Autodesk Inventor part; units mm, degrees
ref_plane "YZ Plane" through (0, 0, 0) normal (1, 0, 0) x (0, 1, 0)
ref_plane "XZ Plane" through (0, 0, 0) normal (0, 1, 0) x (-1, 0, 0)
ref_plane "XY Plane" through (0, 0, 0) normal (0, 0, 1) x (1, 0, 0)
sketch "Sketch1" plane through (0, 0, 0) normal (0, 1, 0) x (-1, 0, 0)
  circle A0 centre (0, 0) radius 6.65
  dimension "d0" = 13.3
extrude "Extrusion1" add sketch "Sketch1" along normal blind 13.3
sketch "Sketch2" plane through (0, 13.3, 0) normal (0, 1, 0) x (1, 0, 0)
  line L0 (0, 10.65) -> (9.2232, 5.325)
  line L1 (9.2232, 5.325) -> (9.2232, -5.325)
  line L2 (9.2232, -5.325) -> (0, -10.65)
  line L3 (0, -10.65) -> (-9.2232, -5.325)
  line L4 (-9.2232, -5.325) -> (-9.2232, 5.325)
  line L5 (-9.2232, 5.325) -> (0, 10.65)
  point P0 (0, 0)
  point P1 (0, 0)
extrude "Extrusion2" add sketch "Sketch2" along normal blind 12.4
sketch "Sketch3" plane through (0, 25.7, 0) normal (0, 1, 0) x (1, 0, 0)
  circle A0 centre (0, 0) radius 11.9
  dimension "d6" = 23.8
extrude "Extrusion3" add sketch "Sketch3" along normal blind 13
sketch "Sketch4" plane through (0, 38.7, 0) normal (0, 1, 0) x (1, 0, 0)
  circle A0 centre (0, 0) radius 11
  dimension "d9" = 22
extrude "Extrusion4" add sketch "Sketch4" along normal blind 1.7
sketch "Sketch5" plane through (0, 40.4, 0) normal (0, 1, 0) x (1, 0, 0)
  circle A0 centre (0, 0) radius 11.9
extrude "Extrusion5" add sketch "Sketch5" along normal blind 4.2
sketch "Sketch6" plane through (0, 44.6, 0) normal (0, 1, 0) x (1, 0, 0)
  circle A0 centre (0, 0) radius 11
extrude "Extrusion6" add sketch "Sketch6" along normal blind 1.8
sketch "Sketch7" plane through (0, 46.4, 0) normal (0, 1, 0) x (1, 0, 0)
  circle A0 centre (0, 0) radius 11.8989
extrude "Extrusion7" add sketch "Sketch7" along normal blind 4.2
sketch "Sketch8" plane through (0, 50.6, 0) normal (0, 1, 0) x (1, 0, 0)
  circle A0 centre (0, 0) radius 11
extrude "Extrusion8" add sketch "Sketch8" along normal blind 2.4
thread "Thread1"
sketch "Sketch9" plane through (0, 53, 0) normal (0, 1, 0) x (1, 0, 0)
  circle A0 centre (0, 0) radius 5.7
  dimension "d22" = 11.4
extrude "Extrusion9" cut sketch "Sketch9" against normal blind 20.6
chamfer "Chamfer1" distance 1 angle 45 1 edges at (-5.7, 53, 0)
sketch "Sketch10" plane through (0, 0, 0) normal (0, -1, 0) x (1, 0, 0)
  circle A0 centre (0, 0) radius 3.75
  dimension "d28" = 7.5
extrude "Extrusion10" cut sketch "Sketch10" against normal blind 29.4
properties part number "AcopleHembra"
Design review of the part built by this model. Coordinates are the model's own, in mm. A direction names the side the tool comes from. Give positions to 0.01 mm unless a question says otherwise; leave off trailing zeros. Loops run counter-clockwise (first coordinate to the right, second up) from the corner with the lowest first, then second, coordinate; pieces in that order, holes last. Notation, with made-up numbers: M 74.25,19.25 L 111.25,19.25 A35 cw 111.25,52.25 Z; hole C 53,87.25 d2. An arc over 180 degrees is marked long. One line per question, with ' | ' between items. Start each with the question number.
1. Add section B-B (y = 48). Write out the cut boundary in (x, z).
2. For faces 1 (the face through (4.547, 19.413, -8.025)), 2 (the face through (-4.68, 19.41, -7.95)), 3 (the face through (0, 13.3, 7)), 4 (the face through (4.68, 19.41, 7.95)), 5 (the face through (3, 38.7, 11)), list the 3-axis set-ups (+Z, -Z, +X, -X, +Y, -Y) from which the entire face can be reached by the end or side of a thin tool; tool diameter is ignored.
3. The part is to be moulded in two halves that separate along Z. For faces 6 (the face through (-4.5, 42.3, 3.5)), 7 (the face through (-4.547, 19.413, 8.025)), 8 (the face through (-3.07, 6.56, 5.9)), say which applies: released by +Z, released by -Z, zero draft, split by the parting line, or undercut.
4. Add section A-A (x = -10.25). Write out the cut boundary in (y, z), plus the area to 3 significant figures.
5. Add section C-C (y = 7). Write out the cut boundary in (x, z).
6. Insertion check: P1, Ø4, axis at y = 40.5, z = -7, coming from the -X side; P2, Ø1, axis at x = 4, z = -8.5, coming from the -Y side; P3, Ø6, axis at y = 11.5, z = -6.5, coming from the +X side. Each pin has a flat end and moves straight along its axis. Give the tip position at first contact, or say it passes through.
7. To check wall thickness, follow L1, parallel to X at y = 46.75, z = 0; L2, parallel to Z at x = 0, y = 23; L3, parallel to Z at x = 0, y = 12.5. State the ranges of each line that lie inside material, in increasing order.
8. Add section D-D (x = -7.25). Write out the cut boundary in (y, z), plus the area to 3 significant figures.
Worked out:
1) outline: C 0,0 d23.8; hole C 0,0 d11.4
2) face 1: -Z, +X, -Y | face 2: -Z, -X, -Y | face 3: -Y | face 4: +Z, +X, -Y | face 5: none
3) face 6: undercut | face 7: released by +Z | face 8: split by the parting line
4) outline: M 25.7,-6.05 L 38.7,-6.05 L 38.7,-3.99 L 40.4,-3.99 L 40.4,-6.05 L 44.6,-6.05 L 44.6,-3.99 L 46.4,-3.99 L 46.4,-6.04 L 50.6,-6.04 L 50.6,-3.99 L 53,-3.99 L 53,3.99 L 50.6,3.99 L 50.6,6.04 L 46.4,6.04 L 46.4,3.99 L 44.6,3.99 L 44.6,6.05 L 40.4,6.05 L 40.4,3.99 L 38.7,3.99 L 38.7,6.05 L 25.7,6.05 Z | area: 306 mm²
5) outline: C 0,0 d13.3; hole C 0,0 d7.5
6) P1: stops at x = -10.8 | P2: stops at y = 13.3 | P3: stops at x = 9.22
7) L1: x = -11.9 to -5.7, 5.7 to 11.9 | L2: z = -10.65 to -3.75, 3.75 to 10.65 | L3: z = -6.65 to -3.75, 3.75 to 6.65
8) outline: M 13.3,-6.46 L 25.7,-6.46 L 25.7,-9.44 L 38.7,-9.44 L 38.7,-8.27 L 40.4,-8.27 L 40.4,-9.44 L 44.6,-9.44 L 44.6,-8.27 L 46.4,-8.27 L 46.4,-9.44 L 50.6,-9.44 L 50.6,-8.27 L 53,-8.27 L 53,8.27 L 50.6,8.27 L 50.6,9.44 L 46.4,9.44 L 46.4,8.27 L 44.6,8.27 L 44.6,9.44 L 40.4,9.44 L 40.4,8.27 L 38.7,8.27 L 38.7,9.44 L 25.7,9.44 L 25.7,6.46 L 13.3,6.46 Z | area: 662 mm²
